Autodesk Inventor part; units mm, degrees
ref_plane "YZ Plane" through (0, 0, 0) normal (1, 0, 0) x (0, 1, 0)
ref_plane "XZ Plane" through (0, 0, 0) normal (0, 1, 0) x (-1, 0, 0)
ref_plane "XY Plane" through (0, 0, 0) normal (0, 0, 1) x (1, 0, 0)
sketch "Sketch1" plane through (0, 0, 0) normal (0, 0, 1) x (1, 0, 0)
  line L0 (0.8, -15.24) -> (-0.8, -15.24)
  line L1 (-0.8, -15.24) -> (-0.8, 15.24)
  line L2 (-0.8, 15.24) -> (0.8, 15.24)
  line L3 (0.8, 15.24) -> (0.8, -15.24)
  line L4 (0.8, -15.24) -> (-0.8, 15.24) construction
  line L5 (-0.8, -15.24) -> (0.8, 15.24) construction
  line L6 (-0.8, -15.24) -> (100.8, -15.24)
  line L7 (100.8, -15.24) -> (100.8, -13.64)
  line L8 (100.8, -13.64) -> (-0.8, -13.64)
  line L9 (-0.8, -13.64) -> (-0.8, -15.24)
  line L10 (-0.8, 15.24) -> (100.8, 15.24)
  line L11 (100.8, 15.24) -> (100.8, 13.64)
  line L12 (100.8, 13.64) -> (-0.8, 13.64)
  line L13 (-0.8, 13.64) -> (-0.8, 15.24)
  line L14 (100.8, -15.24) -> (99.2, -15.24)
  line L15 (99.2, -15.24) -> (99.2, 15.24)
  line L16 (99.2, 15.24) -> (100.8, 15.24)
  line L17 (100.8, 15.24) -> (100.8, -15.24)
  point P0 (0, 0)
  dimension "d0" = 1.6
  dimension "d1" = 30.48
  dimension "d2" = 101.6
  dimension "d3" = 1.6
  dimension "d4" = 101.6
  dimension "d5" = 1.6
  dimension "d6" = 1.6
extrude "Extrusion1" add sketch "Sketch1" along normal blind 19.05 contours L0 L1 L8 L3 | L3 L8 L15 L6 | L8 L1 L12 L3 | L15 L8 L7 L6 | L12 L1 L2 L3 | L3 L10 L15 L12 | L15 L12 L17 L8 | L15 L10 L11 L12
sketch "Sketch2" plane through (-0.8, -15.24, 0) normal (0, -1, 0) x (1, 0, 0)
  line L0 (100, 0) -> (1.6, 0)
  line L1 (0, 0) -> (0, 19.05)
  line L2 (12.78, 0) -> (17.78, 0)
  line L3 (17.78, 0) -> (17.78, 2.4)
  line L4 (17.78, 2.4) -> (12.78, 2.4)
  line L5 (12.78, 2.4) -> (12.78, 0)
  arc A0 (17.78, 2.4) -> (12.78, 2.4) centre (15.28, 2.4) ccw
  point P0 (0.8, 0)
  dimension "d9" = 12.78
  dimension "d10" = 5
  dimension "d11" = 2.4
extrude "Extrusion2" cut sketch "Sketch2" against normal up to surface (30.48 mm away)
ref_plane "Work Plane1" through (50, -15.24, 0) normal (-1, 0, 0) x (0, 0, 1)
sketch "Sketch4" plane through (-0.8, 15.24, 19.05) normal (0, 1, 0) x (1, 0, 0)
  line L0 (12.78, 19.05) -> (17.78, 19.05)
  line L1 (17.78, 19.05) -> (12.78, 19.05)
  line L2 (48.3, 19.05) -> (32.78, 19.05)
  line L3 (32.78, 19.05) -> (32.78, 18.25)
  line L4 (32.78, 18.25) -> (48.3, 18.25)
  line L5 (48.3, 18.25) -> (48.3, 19.05)
  line L6 (17.78, 19.05) -> (17.78, 16.65)
  line L7 (17.78, 19.05) -> (78.82, 19.05)
  line L8 (63.82, 19.05) -> (63.82, 18.25)
  line L9 (63.82, 18.25) -> (48.3, 18.25)
  line L10 (63.82, 19.05) -> (32.78, 19.05)
  line L11 (32.78, 19.05) -> (32.78, 18.25)
  line L12 (32.78, 18.25) -> (63.82, 18.25)
  line L13 (63.82, 18.25) -> (63.82, 19.05)
  point P0 (0.8, 19.05)
  dimension "d15" = 0.8
  dimension "d16" = 15
extrude "Extrusion3" add sketch "Sketch4" against normal up to surface (30.48 mm away)
sketch "Sketch5" plane through (0, 0, 0) normal (0, 0, -1) x (-1, 0, 0)
  line L0 (-99.2, -13.64) -> (-63.02, -13.64)
  line L1 (-99.2, 13.64) -> (-99.2, -13.64)
  line L2 (-63.02, 13.64) -> (-99.2, 13.64)
  line L3 (-63.02, 13.64) -> (-63.02, -13.64)
  line L4 (-31.98, 13.64) -> (-31.98, -13.64)
  line L5 (-16.98, 13.64) -> (-31.98, 13.64)
  line L6 (-16.98, 13.64) -> (-16.98, 15.24)
  line L7 (-100.8, 15.24) -> (-16.98, 15.24)
  line L8 (-100.8, -15.24) -> (-100.8, 15.24)
  line L9 (-16.98, -15.24) -> (-100.8, -15.24)
  line L10 (-16.98, -15.24) -> (-16.98, -13.64)
  line L11 (-31.98, -13.64) -> (-16.98, -13.64)
  line L12 (-11.98, -13.64) -> (-11.98, -15.24)
  line L13 (0.8, -15.24) -> (-11.98, -15.24)
  line L14 (0.8, 15.24) -> (0.8, -15.24)
  line L15 (-11.98, 15.24) -> (0.8, 15.24)
  line L16 (-11.98, 15.24) -> (-11.98, 13.64)
  line L17 (-0.8, 13.64) -> (-11.98, 13.64)
  line L18 (-0.8, -13.64) -> (-0.8, 13.64)
  line L19 (-11.98, -13.64) -> (-0.8, -13.64)
  line L20 (-100.8, -15.24) -> (-31.966, -15.24)
  line L21 (-31.966, -15.24) -> (-31.966, -17.094)
  line L22 (-31.966, -17.094) -> (-100.8, -17.094)
  line L23 (-100.8, -17.094) -> (-100.8, -15.24)
  point P0 (0, 0)
  dimension "d19" = 32.766
  dimension "d20" = 17.094
extrude "Extrusion4" add sketch "Sketch5" against normal up to surface (19.05 mm away) contours L21 L22 L23 L9
sketch "Sketch6" plane through (0, 0, 19.05) normal (0, 0, 1) x (1, 0, 0)
  line L0 (100.8, 15.24) -> (100.8, -17.094)
  line L1 (100.8, 15.24) -> (-0.8, 15.24)
  line L2 (-0.8, 15.24) -> (-0.8, -15.24)
  line L3 (-0.8, -15.24) -> (31.966, -15.24)
  line L4 (31.966, -17.094) -> (31.966, -15.24)
  line L5 (100.8, -17.094) -> (31.966, -17.094)
  line L6 (99.2, 13.64) -> (99.2, -13.64)
  line L7 (99.2, -13.64) -> (0.8, -13.64)
  line L8 (0.8, -13.64) -> (0.8, 13.64)
  line L9 (0.8, 13.64) -> (99.2, 13.64)
  line L10 (99.2, -13.64) -> (33.566, -13.64)
  line L11 (33.566, -13.64) -> (33.566, -15.494)
  line L12 (33.566, -15.494) -> (99.2, -15.494)
  line L13 (99.2, -15.494) -> (99.2, -13.64)
  point P0 (0, 0)
  dimension "d23" = 1.6
  dimension "d24" = 1.6
extrude "Extrusion5" cut sketch "Sketch6" against normal up to surface (18.25 mm away) contours L13 L12 L11 L7
mirror "Mirror3" about plane through (0, 0, 0) normal (0, 1, 0) of "Extrusion4", "Extrusion5"
sketch "Sketch7" plane through (63.02, -13.64, 0) normal (1, 0, 0) x (0, 0, -1)
  line L0 (0, 0) -> (-0.8, 0)
  line L1 (0, 27.28) -> (0, 0)
  line L2 (-0.8, 27.28) -> (0, 27.28)
  line L3 (-0.8, 27.28) -> (-0.8, 0)
  point P0 (0, 13.64)
extrude "Extrusion6" add sketch "Sketch7" along normal up to next
properties part number "CarChassis"
The listing builds one solid part. Answer for the finished solid, in the listing's coordinates (mm). A direction names the side the tool comes from. Coordinates: 2 decimals unless noted, no trailing zeros. Write each loop counter-clockwise with the first axis right and the second up, starting at its lowest first coordinate (ties: lowest second). Pieces come first, ordered by that corner, then holes.
Q1. Given P1, Ø15.5, axis at x = 76, y = 7, coming from the +Z side; P2, Ø9.5, axis at x = 23, z = 13, coming from the +Y side; P3, Ø5.5, axis at x = 16.5, z = 12, coming from the -Y side, each flat-ended and moving along its own axis, determine where each tip first touches the part or whether it passes through.
Returned:
P1: stops at z = 0.8
P2: stops at y = 15.24
P3: stops at y = -15.24
Q2. The mould has two halves that part along X. Classify faces 4 (the flat face through (100.8, 0, 9)), 5 (the flat face through (0.8, 0, 9)), 6 (the flat face through (67, 17.094, 9)): released by +X, released by -X, zero draft, split by the parting line, or undercut.
Returned:
face 4: released by +X
face 5: undercut
face 6: zero draft
Q3. Section B-B, the plane y = 2 is taken. Write down the section's boundary in (x, z).
Returned:
outline: (-0.8, 0) - (0.8, 0) - (0.8, 19.05) - (-0.8, 19.05) - close; (31.98, 0) - (100.8, 0) - (100.8, 19.05) - (99.2, 19.05) - (99.2, 0.8) - (31.98, 0.8) - close
Q4. Section C-C, the plane z = 16.5 is taken. Write down the section's boundary in (x, y), then the cut area to 3 significant figures.
Returned:
outline: (-0.8, -15.24) - (31.97, -15.24) - (31.97, -17.09) - (100.8, -17.09) - (100.8, 17.09) - (31.97, 17.09) - (31.97, 15.24) - (-0.8, 15.24) - close; hole (0.8, -13.64) - (33.57, -13.64) - (33.57, -15.49) - (99.2, -15.49) - (99.2, 15.49) - (33.57, 15.49) - (33.57, 13.64) - (0.8, 13.64) - close
area: 424 mm2
Q5. Which of the six approach directions +Z, -Z, +X, -X, +Y, -Y give full straight-line access (tool end or side, diameter ignored) to faces 1 (the flat face through (31.966, -16, 9)), 2 (the flat face through (15, 15.24, 9)), 3 (the flat face through (33.566, -15, 10))?
Returned:
face 1: +Z, -Z, -X, -Y
face 2: +Z, -Z, -X, +Y
face 3: +Z
Q6. Section A-A, the plane x = 22.5 is taken. Write down the section's boundary in (y, z).
Returned:
outline: (-15.24, 0) - (-13.64, 0) - (-13.64, 19.05) - (-15.24, 19.05) - close; (13.64, 0) - (15.24, 0) - (15.24, 19.05) - (13.64, 19.05) - close
Q7. Find the intervals of material crossed by line 1 along Y through (x, z) = (50, 17.5); line 2 along Y through (x, z) = (13, 18); line 3 along X through (y, z) = (12.5, 12.5), in increasing order.
Returned:
line 1: y = -17.09 to -15.49, 15.49 to 17.09
line 2: y = -15.24 to -13.64, 13.64 to 15.24
line 3: x = -0.8 to 0.8, 99.2 to 100.8
Q8. Section D-D, the plane x = 80 is taken. Write down the section's boundary in (y, z), then the cut area to 3 significant figures.
Returned:
outline: (-17.09, 0) - (17.09, 0) - (17.09, 19.05) - (15.49, 19.05) - (15.49, 0.8) - (-15.49, 0.8) - (-15.49, 19.05) - (-17.09, 19.05) - close
area: 85.8 mm2
